Read the model definition and answer for the solid it produces. Units are mm, in the model's axes. A direction names the side the tool comes from. Coordinates: 2 decimals unless noted, no trailing zeros. Order: outer loops, then holes, each group sorted by start corner. A loop starts at its lowest first (then second) coordinate and runs counter-clockwise, first axis right, second up.
```python
from build123d import *

# Parameters (mm, degrees)
F1_DEPTH  = 98.425
F2_W      = 25.4
F2_H      = 25.4
F2_H_2    = 29.21
F3_DEPTH  = 50.801
F4_W      = 25.4
F4_H      = 29.21
F5_DEPTH  = 3.175
F6_W      = 6.35
F6_H      = 2.54
F7_DEPTH  = 12.7
F8_W      = 9.525
F8_H      = 2.54
F9_DEPTH  = 12.7
F10_W     = 190.5
F10_H     = 27.94
F11_DEPTH = 3.175


with BuildPart() as f1:
    # F0 (on Right) → F1 (new body, symmetric)
    with BuildSketch(Plane.YZ):
        Polygon((-66.675, 0), (0, 0), (0, 50.8), (-31.75, 50.8), (-31.75, 31.75), (-66.675, 31.75), align=None)
    extrude(amount=F1_DEPTH, both=True)

    # F2 (on face) → F3 (cut, through all)
    with BuildSketch(Plane(origin=(0, 0, 0), x_dir=(1, 0, 0), z_dir=(0, 0, -1))):
        with Locations((-15.875, 51.435)):
            Rectangle(F2_W, F2_H)
        with Locations((-15.875, 17.145)):
            Rectangle(F2_W, F2_H_2)
        with Locations((-47.625, 17.145)):
            Rectangle(F2_W, F2_H_2)
        with Locations((-47.625, 51.435)):
            Rectangle(F2_W, F2_H)
        with Locations((-79.375, 17.145)):
            Rectangle(F2_W, F2_H_2)
        with Locations((-79.375, 51.435)):
            Rectangle(F2_W, F2_H)
        with Locations((47.625, 17.145)):
            Rectangle(F2_W, F2_H_2)
        with Locations((15.875, 51.435)):
            Rectangle(F2_W, F2_H)
        with Locations((79.375, 17.145)):
            Rectangle(F2_W, F2_H_2)
        with Locations((47.625, 51.435)):
            Rectangle(F2_W, F2_H)
        with Locations((79.375, 51.435)):
            Rectangle(F2_W, F2_H)
        with Locations((15.875, 17.145)):
            Rectangle(F2_W, F2_H_2)
    extrude(amount=-F3_DEPTH, mode=Mode.SUBTRACT)

    # F4 (on face) → F5 (join)
    with BuildSketch(Plane.XY.offset(31.75)):
        with Locations((15.875, -17.145)):
            Rectangle(F4_W, F4_H)
        with Locations((47.625, -17.145)):
            Rectangle(F4_W, F4_H)
        with Locations((79.375, -17.145)):
            Rectangle(F4_W, F4_H)
        with Locations((-15.875, -17.145)):
            Rectangle(F4_W, F4_H)
        with Locations((-79.375, -17.145)):
            Rectangle(F4_W, F4_H)
        with Locations((-47.625, -17.145)):
            Rectangle(F4_W, F4_H)
    extrude(amount=-F5_DEPTH)

    # F6 (on face) → F7 (join)
    with BuildSketch(Plane.XY.offset(31.75)):
        with Locations((-88.9, -30.48)):
            Rectangle(F6_W, F6_H)
        with Locations((-69.85, -30.48)):
            Rectangle(F6_W, F6_H)
        with Locations((-38.1, -30.48)):
            Rectangle(F6_W, F6_H)
        with Locations((-57.15, -30.48)):
            Rectangle(F6_W, F6_H)
        with Locations((-6.35, -30.48)):
            Rectangle(F6_W, F6_H)
        with Locations((-25.4, -30.48)):
            Rectangle(F6_W, F6_H)
        with Locations((25.4, -30.48)):
            Rectangle(F6_W, F6_H)
        with Locations((6.35, -30.48)):
            Rectangle(F6_W, F6_H)
        with Locations((57.15, -30.48)):
            Rectangle(F6_W, F6_H)
        with Locations((38.1, -30.48)):
            Rectangle(F6_W, F6_H)
        with Locations((88.9, -30.48)):
            Rectangle(F6_W, F6_H)
        with Locations((69.85, -30.48)):
            Rectangle(F6_W, F6_H)
    extrude(amount=F7_DEPTH)

    # F8 (on face) → F9 (cut)
    with BuildSketch(Plane.XY.offset(31.75)):
        with Locations((-79.375, -65.405)):
            Rectangle(F8_W, F8_H)
        with Locations((-47.625, -65.405)):
            Rectangle(F8_W, F8_H)
        with Locations((-15.875, -65.405)):
            Rectangle(F8_W, F8_H)
        with Locations((15.875, -65.405)):
            Rectangle(F8_W, F8_H)
        with Locations((47.625, -65.405)):
            Rectangle(F8_W, F8_H)
        with Locations((79.375, -65.405)):
            Rectangle(F8_W, F8_H)
    extrude(amount=-F9_DEPTH, mode=Mode.SUBTRACT)

    # F10 (on face) → F11 (join)
    with BuildSketch(Plane(origin=(0, 0, 0), x_dir=(1, 0, 0), z_dir=(0, 0, -1))):
        with Locations((-3.175, 52.705)):
            Rectangle(F10_W, F10_H)
    extrude(amount=-F11_DEPTH)


solid = f1.part
```
1) A cutting plane is placed at C-C, the plane x = -6.5. Determine the outline of the cut face in (y, z) (3 decimals).
A:
outline: (-66.675, 0) - (-31.75, 0) - (-31.75, 28.575) - (-2.54, 28.575) - (-2.54, 0) - (0, 0) - (0, 50.8) - (-2.54, 50.8) - (-2.54, 31.75) - (-29.21, 31.75) - (-29.21, 44.45) - (-31.75, 44.45) - (-31.75, 31.75) - (-38.735, 31.75) - (-38.735, 3.175) - (-64.135, 3.175) - (-64.135, 31.75) - (-66.675, 31.75) - close
2) A cutting plane is placed at B-B, the plane y = -55.5. Determine the outline of the cut face in (x, z) (3 decimals), and give its area (3 significant figures).
A:
outline: (-98.425, 0) - (98.425, 0) - (98.425, 31.75) - (92.075, 31.75) - (92.075, 3.175) - (66.675, 3.175) - (66.675, 31.75) - (60.325, 31.75) - (60.325, 3.175) - (34.925, 3.175) - (34.925, 31.75) - (28.575, 31.75) - (28.575, 3.175) - (3.175, 3.175) - (3.175, 31.75) - (-3.175, 31.75) - (-3.175, 3.175) - (-28.575, 3.175) - (-28.575, 31.75) - (-34.925, 31.75) - (-34.925, 3.175) - (-60.325, 3.175) - (-60.325, 31.75) - (-66.675, 31.75) - (-66.675, 3.175) - (-92.075, 3.175) - (-92.075, 31.75) - (-98.425, 31.75) - close
area: 1,900 mm2
3) Determine the mould class of faces 1 (the flat face through (1, -66.675, 16)), 2 (the flat face through (16, -38.735, 17)) for opening direction X: pulls with the +X half, pulls with the -X half, needs draft (parallel to the pull), parting line crosses it, or undercut.
A:
face 1: needs draft
face 2: undercut
4) A cutting plane is placed at A-A, the plane z = 47.5. Determine the outline of the cut face in (x, y) (3 decimals).
A:
outline: (-98.425, -31.75) - (-92.075, -31.75) - (-92.075, -2.54) - (-66.675, -2.54) - (-66.675, -31.75) - (-60.325, -31.75) - (-60.325, -2.54) - (-34.925, -2.54) - (-34.925, -31.75) - (-28.575, -31.75) - (-28.575, -2.54) - (-3.175, -2.54) - (-3.175, -31.75) - (3.175, -31.75) - (3.175, -2.54) - (28.575, -2.54) - (28.575, -31.75) - (34.925, -31.75) - (34.925, -2.54) - (60.325, -2.54) - (60.325, -31.75) - (66.675, -31.75) - (66.675, -2.54) - (92.075, -2.54) - (92.075, -31.75) - (98.425, -31.75) - (98.425, 0) - (-98.425, 0) - close
5) Flat-ended cylindrical pins translate along their axes: pin 1 Ø9.5 at (x, z) = (53, 43.5) entering from -Y; pin 2 Ø2 at (x, y) = (79.5, -66) entering from +Z; pin 3 Ø5 at (y, z) = (-55, 36) entering from -X; pin 4 Ø12.5 at (x, y) = (75.5, -14) entering from -Z (3 decimals). Find the tip coordinate at first contact, or state that the pin passes through.
A:
pin 1: stops at y = -31.75
pin 2: stops at z = 19.05
pin 3: passes through
pin 4: stops at z = 28.575
6) Straight lines are drawn through the part: line 1 (Y direction, x = 57, z = 6.5) (3 decimals); line 2 (Y direction, x = 38, z = 39.5); line 3 (Y direction, x = 48, z = 24.5) (3 decimals). For each, find the intervals that lie inside material, in ascending order.
A:
line 1: y = -66.675 to -64.135, -38.735 to -31.75, -2.54 to 0
line 2: y = -31.75 to -29.21, -2.54 to 0
line 3: y = -38.735 to -31.75, -2.54 to 0
7) Which of the six approach directions +Z, -Z, +X, -X, +Y, -Y give full straight-line access (tool end or side, diameter ignored) to faces 3 (the flat face through (-25, -29.21, 38)), 4 (the flat face through (-48, -2.54, 14)), 5 (the flat face through (0, -31.75, 39))?
A:
face 3: +Z
face 4: -Z
face 5: +Z, +X, -X, -Y
8) A cutting plane is placed at D-D, the plane z = 5. State how many separate pieces and enclosed holes the cut face has, and give its area (3 significant figures).
A:
separate pieces: 1
enclosed holes: 12
area: 4,800 mm2
